from build123d import *

# Parameters (mm, degrees)
SKETCH1_R                  = 9
SKETCH1_R_2                = 6
MAIN_DEPTH                 = 9.5
SKETCH2_W                  = 25
SKETCH2_H                  = 19
SKETCH2_R                  = 4
SKETCH2_R_2                = 1.35
BALLSUPPORTEXTRUSION_DEPTH = 2.5
SKETCH3_R                  = 5.15
BALLSUPPORTHOLE_DEPTH      = 4
FILLET2_R                  = 2
SKETCH5_R                  = 6
CUT_EXTRUDE2_DEPTH         = 20


with BuildPart() as part:
    # Sketch1 → Main (new body, symmetric)
    with BuildSketch(Plane.XY):
        Circle(SKETCH1_R)
        Circle(SKETCH1_R_2, mode=Mode.SUBTRACT)
    extrude(amount=MAIN_DEPTH, both=True)

    # Sketch2 → BallSupportExtrusion (add, symmetric)
    with BuildSketch(Plane(origin=(0, 0, 0), x_dir=(1, 0, 0), z_dir=(0, 1, 0))):
        with Locations((12.5, 0)):
            Rectangle(SKETCH2_W, SKETCH2_H)
        with Locations((18, 0)):
            Circle(SKETCH2_R, mode=Mode.SUBTRACT)
        with Locations((18, 7)):
            Circle(SKETCH2_R_2, mode=Mode.SUBTRACT)
        with Locations((18, -7)):
            Circle(SKETCH2_R_2, mode=Mode.SUBTRACT)
    extrude(amount=BALLSUPPORTEXTRUSION_DEPTH, both=True)

    # Sketch3 → BallSupportHole (cut)
    with BuildSketch(Plane(origin=(0, 2.5, 0), x_dir=(1, 0, 0), z_dir=(0, 1, 0))):
        with Locations((18, 0)):
            Circle(SKETCH3_R)
    extrude(amount=-BALLSUPPORTHOLE_DEPTH, mode=Mode.SUBTRACT)

    # Fillet2
    fillet2_edges = [part.edges().sort_by_distance(p)[0] for p in [
        (8.645808233, 2.5, 0),
    ]]
    fillet(fillet2_edges, radius=FILLET2_R)

    # Sketch5 → Cut-Extrude2 (cut, through all)
    with BuildSketch(Plane.XY.offset(9.5)):
        Circle(SKETCH5_R)
    extrude(amount=-CUT_EXTRUDE2_DEPTH, mode=Mode.SUBTRACT)


solid = part.part
Input: part model. Units: mm. Frame: model coordinates. A direction names the side the tool comes from. Coordinates: 2 decimals unless noted, no trailing zeros. Loops run counter-clockwise (first coordinate to the right, second up) from the corner with the lowest first, then second, coordinate; pieces in that order, holes last. Notation, with made-up numbers: (-30, 73.5) -> (-26, 73.5) arc R17 ccw to (-26, 99.5) -> close; hole circle Ø4 at (27, 53). An arc over 180 degrees is marked (long way). Write each question's results on one line, items separated by ' | '. Start each with the question number.
Q1. Section A-A, the plane z = 0. Return the cut outline in (x, y).
Q2. Pull-direction query (Z, two-part tool) for faces 4 (the cylindrical face through (-6, 0, 0)), 5 (the flat face through (8, 0, -9.5)), 6 (the cylindrical face through (14, -2, 0)); classes: released by +Z, released by -Z, zero draft, split by the parting line, or undercut.
Q3. Reachability of faces 1 (the flat face through (13, -2.5, 0)), 2 (the flat face through (21, -1.5, 3)), 3 (the flat face through (12, 2.5, 0)) from +Z, -Z, +X, -X, +Y, -Y: full face, straight path, thin tool, end or side. Return the list, or none.
Q4. Ray query, line 1 (Z direction, x = 18, y = 0.6); line 2 (Z direction, x = 18, y = -2.2); line 3 (Y direction, x = 0, z = -0.25). Return the intervals inside material, ascending. Write a range as from..to.
Q5. Section D-D, the plane x = 18. Return the cut outline in (y, z), plus the area to 3 significant figures.
Q6. Section B-B, the plane x = 0. Return the cut outline in (y, z).
Q7. Pin query (flat end, axial travel): pin 1 (10.5 mm diameter, centred on x = 18, z = 0, fed in from +Y); pin 2 (4.5 mm diameter, centred on x = 18, z = -7, fed in from -Y); pin 3 (10 mm diameter, centred on y = -2, z = 7.5, fed in from -X); pin 4 (9.5 mm diameter, centred on x = 18, z = 0, fed in from +Y). Return the tip coordinate at first contact, or that it passes through.
Q8. Section C-C, the plane y = 0. Return the cut outline in (x, z), plus the area to 3 significant figures.
Found:
1) outline: (8.21, 3.68) arc R9 ccw (long way) to (8.65, -2.5) -> (14, -2.5) -> (14, -1.5) -> (12.85, -1.5) -> (12.85, 2.5) -> (10.04, 2.5) arc R2 cw to start; (22, -2.5) -> (25, -2.5) -> (25, 2.5) -> (23.15, 2.5) -> (23.15, -1.5) -> (22, -1.5) -> close; hole circle Ø12 at (0, 0)
2) face 4: zero draft | face 5: released by -Z | face 6: undercut
3) face 1: +Z, -Z, +X, -Y | face 2: +Y | face 3: +Z, -Z, +X, +Y
4) line 1: -9.5..-8.35, -5.65..-5.15, 5.15..5.65, 8.35..9.5 | line 2: -9.5..-8.35, -5.65..-4, 4..5.65, 8.35..9.5 | line 3: -9..-6, 6..9
5) outline: (-2.5, -9.5) -> (2.5, -9.5) -> (2.5, -8.35) -> (-2.5, -8.35) -> close; (-2.5, -5.65) -> (2.5, -5.65) -> (2.5, -5.15) -> (-1.5, -5.15) -> (-1.5, -4) -> (-2.5, -4) -> close; (-2.5, 4) -> (-1.5, 4) -> (-1.5, 5.15) -> (2.5, 5.15) -> (2.5, 5.65) -> (-2.5, 5.65) -> close; (-2.5, 8.35) -> (2.5, 8.35) -> (2.5, 9.5) -> (-2.5, 9.5) -> close | area: 18.8 mm2
6) outline: (-9, -9.5) -> (-6, -9.5) -> (-6, 9.5) -> (-9, 9.5) -> close; (6, -9.5) -> (9, -9.5) -> (9, 9.5) -> (6, 9.5) -> close
7) pin 1: y = 2.5 | pin 2: y = -2.5 | pin 3: x = -9 | pin 4: y = -1.5
8) outline: (-9, -9.5) -> (-6, -9.5) -> (-6, 9.5) -> (-9, 9.5) -> close; (6, -9.5) -> (25, -9.5) -> (25, 9.5) -> (6, 9.5) -> close; hole circle Ø10.3 at (18, 0); hole circle Ø2.7 at (18, -7); hole circle Ø2.7 at (18, 7) | area: 323 mm2
